```python
from build123d import *

# Parameters (mm, degrees)
BOSS_EXTRUDE1_DEPTH = 8
CIRPATTERN1_COUNT   = 14
CIRPATTERN1_ANGLE   = 332.8
SKETCH3_R           = 4
CUT_EXTRUDE2_DEPTH  = 2
SKETCH2_R           = 2.85
CUT_EXTRUDE4_DEPTH  = 14


with BuildPart() as part:
    # Sketch1 → Boss-Extrude1 (new body)
    with BuildSketch(Plane.XY):
        with BuildLine():
            Line((-1, 18), (1, 18))
            add(Edge.make_bspline(
                [(1, 18), (1.578443342, 17.032357733), (1.90693166, 15.988363393), (1.985464954, 14.86801698)],
                knots=[0, 0, 0, 0, 0.922231511, 0.922231511, 0.922231511, 0.922231511], degree=3))
            ThreePointArc((1.985464954, 14.86801698), (0.003612333, -14.999999565), (-1.99262582, 14.867058967))
            add(Edge.make_bspline(
                [(-1, 18), (-1.608825246, 17.079975603), (-1.93970052, 16.035661926), (-1.99262582, 14.867058967)],
                knots=[0, 0, 0, 0, 0.925626866, 0.925626866, 0.925626866, 0.925626866], degree=3))
        make_face()
    boss_extrude1 = extrude(amount=BOSS_EXTRUDE1_DEPTH)

    # CirPattern1: Boss-Extrude1 ×14 about axis
    cirpattern1_axis = Axis((0, 0, 8), (0, 0, -1))
    for i in range(1, CIRPATTERN1_COUNT):
        add(boss_extrude1.rotate(cirpattern1_axis, i * CIRPATTERN1_ANGLE / (CIRPATTERN1_COUNT - 1)))

    # Sketch3 → Cut-Extrude2 (cut)
    with BuildSketch(Plane.XY.offset(8)):
        Circle(SKETCH3_R)
    extrude(amount=-CUT_EXTRUDE2_DEPTH, mode=Mode.SUBTRACT)

    # Sketch2 → Cut-Extrude4 (cut)
    with BuildSketch(Plane.XY.offset(8)):
        Circle(SKETCH2_R)
    extrude(amount=-CUT_EXTRUDE4_DEPTH, mode=Mode.SUBTRACT)


solid = part.part
```
Read the model definition and answer for the solid it produces. Units are mm, in the model's axes. A direction names the side the tool comes from. Give positions to 0.01 mm unless a question says otherwise; leave off trailing zeros. Write each loop counter-clockwise with the first axis right and the second up, starting at its lowest first coordinate (ties: lowest second). Pieces come first, ordered by that corner, then holes. Notation, with made-up numbers: (59, -34.75) - (78, -34.75) arc R20 cw to (78, -17.75) - close; hole circle Ø2 at (-27.5, 39.25). An arc over 180 degrees is marked (long way). Write item = value, one per line. Start each with the question number.
Item 1: A tool of negligible diameter and unlimited length cuts with its end or side. For faces 5 (the cylindrical face through (-9.659, 11.476, 3.944)), 6 (the flat face through (14.193, -11.071, 3.944)), from which of +Z, -Z, +X, -X, +Y, -Y can it reach the whole face along a straight path? Write none if from no direction.
Item 2: Find the intervals of material crossed by probe 1 along Y at (x, z) = (0, 2.5); probe 2 along Y at (x, z) = (0, 7.15); probe 3 along X at (y, z) = (-0.5, 5), in increasing order. Write a range as [from, to].
Item 3: Find section B-B (x = 0). Give the vertices of the cut face in (y, z).
Item 4: Find section A-A (y = 0). Give the vertices of the cut face in (x, z), then the cut area to 3 significant figures.
Item 5: The mould has two halves that part along X. Classify faces 1 (the flat face through (14.02, 11.29, 3.94)), 2 (the cylindrical face through (3.549, -14.574, 3.944)), 3 (the flat face through (2, -3, 0)), 4 (the flat face through (-1, 3, 6)): +X half, -X half, draft (parallel to the pull), parting line (faces both ways), or undercut.
Item 6: Each of these flat-tipped pins is pushed along its axis until it touches: P1, Ø1, axis at x = -10.5, z = 6, coming from the -Y side; P2, Ø2, axis at y = 8, z = 6.5, coming from the -X side; P3, Ø4, axis at x = 4, z = 3.5, coming from the +Y side. Where does it stop, or does it pass through?
Response:
q1.face_5 = +Z, -Z
q1.face_6 = +Z, -Z, +X, -Y
q2.probe_1 = [-18, -2.85], [2.85, 18]
q2.probe_2 = [-18, -4], [4, 18]
q2.probe_3 = [-14.99, -2.81], [2.81, 14.99]
q3.outline = (-18, 0) - (-2.85, 0) - (-2.85, 6) - (-4, 6) - (-4, 8) - (-18, 8) - close; (2.85, 0) - (18, 0) - (18, 8) - (4, 8) - (4, 6) - (2.85, 6) - close
q4.outline = (-15, 0) - (-2.85, 0) - (-2.85, 6) - (-4, 6) - (-4, 8) - (-15, 8) - close; (2.85, 0) - (15, 0) - (15, 8) - (4, 8) - (4, 6) - (2.85, 6) - close
q4.area = 190 mm²
q5.face_1 = +X half
q5.face_2 = undercut
q5.face_3 = draft
q5.face_4 = undercut
q6.P1 = -11.54
q6.P2 = -14.43
q6.P3 = 16.03
